Here's how the part is built. I have some questions about the finished solid (model axes, mm). A direction names the side the tool comes from. Round coordinates to 2 decimals unless told otherwise and drop trailing zeros. Loops run counter-clockwise (first coordinate to the right, second up) from the corner with the lowest first, then second, coordinate; pieces in that order, holes last. Notation, with made-up numbers: M 0,16 L 40,16 A22 cw 40,35 Z; hole C 14,-9 d1. An arc over 180 degrees is marked long. Answer as a JSON object with one key per item and string values.
from build123d import *

# Parameters (mm, degrees)
F0_R     = 44.45
F1_DEPTH = 76.2
F2_R     = 25.4
F3_W     = 88.9
F3_H     = 76.2
F4_DEPTH = 38.1


with BuildPart() as f1:
    # F0 (on Top) → F1 (new body)
    with BuildSketch(Plane.XY):
        with Locations((0, 21.087829)):
            Circle(F0_R)
    extrude(amount=F1_DEPTH)

    # F2
    f2_edges = [f1.edges().sort_by_distance(p)[0] for p in [
        (-44.45, 21.087829, 76.2),
    ]]
    fillet(f2_edges, radius=F2_R)

    # F3 (on Top) → F4 (join)
    with BuildSketch(Plane.XY):
        with Locations((-0.375016, -38.1)):
            Rectangle(F3_W, F3_H)
        with Locations((-0.375016, 85.672979)):
            Rectangle(F3_W, F3_H)
    extrude(amount=F4_DEPTH)


solid = f1.part
Item 1: I want a section at A-A on z = 8. List the corners of the cut face in (x, y) for me, plus the area to 3 significant figures.
Solution:
{"outline": "M -44.83,-76.2 L 44.07,-76.2 L 44.07,0 L 39.13,0 A44.45 ccw 35.7,47.57 L 44.07,47.57 L 44.07,123.77 L -44.83,123.77 L -44.83,47.57 L -35.7,47.57 A44.45 ccw -39.13,0 L -44.83,0 Z", "area": "17,600 mm2"}
Item 2: For P1, Ø5, axis at x = 11.5, y = 44, coming from the -Z side; P2, Ø3, axis at y = 101.5, z = 37, coming from the +X side (3 decimals); P3, Ø23, axis at x = -12, y = 83.5, coming from the +Z side; P4, Ø2, axis at x = 14.5, y = 58.5, coming from the +Z side, each with a flat end and sliding along its axis, tell me the tip position at first contact or that it passes through.
Solution:
{"P1": "stops at z = 0", "P2": "stops at x = 44.075", "P3": "stops at z = 38.1", "P4": "stops at z = 66.36"}
Item 3: For faces 5 (the face through (44.075, -39, 19)), 6 (the face through (0, 21, 76.2)), 7 (the face through (44.075, 85, 19)), which set-ups out of +Z, -Z, +X, -X, +Y, -Y let a thin tool reach every point of the face, with its end or its side?
Solution:
{"face 5": "+Z, -Z, +X, -Y", "face 6": "+Z, +X, -X, +Y, -Y", "face 7": "+Z, -Z, +X, +Y"}
Item 4: We'd pull the mould along Y, two halves only. Please class faces 1 (the face through (-1, -76.2, 19)), 2 (the face through (-40, 47.573, 19)), 3 (the face through (-44.825, 85, 19)), 4 (the face through (-1, 123.773, 19)): +Y half, -Y half, draft (parallel to the pull), parting line (faces both ways), or undercut.
Solution:
{"face 1": "-Y half", "face 2": "undercut", "face 3": "draft", "face 4": "+Y half"}
Item 5: If I drill on L1, parallel to Z at x = 11.5, y = 110.5; L2, parallel to X at y = 114.5, z = 14.5; L3, parallel to Y at x = -1.5, z = 65.5, over which ranges is the centre line in solid material (lowest first)? Write a range as from..to.
Solution:
{"L1": "z = 0..38.1", "L2": "x = -44.83..44.07", "L3": "y = -18.65..60.82"}
Item 6: I want a section at B-B on y = 102. List the corners of the cut face in (x, z) for me.
Solution:
{"outline": "M -44.83,0 L 44.07,0 L 44.07,38.1 L -44.83,38.1 Z"}
Item 7: I want a section at C-C on z = 40.5. List the corners of the cut face in (x, y) for me.
Solution:
{"outline": "C 0,21.09 d88.9"}
